```python
from build123d import *

# Parameters (mm, degrees)
EXTRUDE_1_DEPTH     = 20
REVOLVE_1_ANGLE     = 180
CUT_EXTRUDE_START   = -19
CUT_EXTRUDE_1_DEPTH = 19
SKETCH_5_R          = 10
CUT_EXTRUDE_2_DEPTH = 87.442177205
SKETCH_4_R          = 1.25
SKETCH_4_R_2        = 5.1
CUT_EXTRUDE_3_DEPTH = 86.97819491
CUT_EXTRUDE_START_2 = -3
CUT_EXTRUDE_5_DEPTH = 3
SKETCH_6_R          = 6
CUT_EXTRUDE_4_DEPTH = 4.2
CUT_EXTRUDE_6_DEPTH = 5
HOLE_WIZARD_1_D     = 1.7
HOLE_WIZARD_1_DEPTH = 3.5
CHAMFER_1_SIZE      = 0.3


with BuildPart() as part:
    # 草图2 → 凸台-拉伸1 (new body)
    with BuildSketch(Plane(origin=(0, 0, 0), x_dir=(1, 0, 0), z_dir=(0, 1, 0))):
        with BuildLine():
            Line((70.446428571, 12.492025518), (0.535714286, 14.990430621))
            ThreePointArc((0.535714286, 14.990430621), (-10.415476122, 10.794343757), (-15, 0))
            Line((-15, 0), (82.5, 0))
            ThreePointArc((82.5, 0), (78.995286464, 8.679563435), (70.446428571, 12.492025518))
        make_face()
        with BuildLine():
            Line((82.5, 0), (-15, 0))
            ThreePointArc((-15, 0), (-10.415476122, -10.794343757), (0.535714286, -14.990430621))
            Line((0.535714286, -14.990430621), (70.446428571, -12.492025518))
            ThreePointArc((70.446428571, -12.492025518), (78.995286464, -8.679563435), (82.5, 0))
        make_face()
    extrude(amount=EXTRUDE_1_DEPTH)

    # 草图1 → 旋转1 (revolve)
    with BuildSketch(Plane(origin=(0, 0, 0), x_dir=(1, 0, 0), z_dir=(0, 1, 0))):
        with BuildLine():
            Line((0.535714286, -14.990430621), (70.446428571, -12.492025518))
            ThreePointArc((70.446428571, -12.492025518), (78.995286464, -8.679563435), (82.5, 0))
            Line((82.5, 0), (-15, 0))
            ThreePointArc((-15, 0), (-10.415476122, -10.794343757), (0.535714286, -14.990430621))
        make_face()
    revolve(axis=Axis((70, 0, 0), (1, 0, 0)), revolution_arc=REVOLVE_1_ANGLE)

    # 草图3 → 切除-拉伸1 (cut)
    with BuildSketch(Plane(origin=(0, 20, 0), x_dir=(1, 0, 0), z_dir=(0, 1, 0)).offset(CUT_EXTRUDE_START)):
        with BuildLine():
            Line((17.295525226, 14.391483841), (0.535714286, 14.990430621))
            ThreePointArc((0.535714286, 14.990430621), (-15, 0), (0.535714286, -14.990430621))
            Line((0.535714286, -14.990430621), (17.295525226, -14.391483841))
            ThreePointArc((17.295525226, -14.391483841), (22.5, 0), (17.295525226, 14.391483841))
        make_face()
    extrude(amount=CUT_EXTRUDE_1_DEPTH, mode=Mode.SUBTRACT)

    # 草图5 → 切除-拉伸2 (cut, through all)
    with BuildSketch(Plane(origin=(0, -1, 0), x_dir=(1, 0, 0), z_dir=(0, 1, 0))):
        with Locations(Location((0, 0, 0), (0, 0, 270))):
            Circle(SKETCH_5_R)
    extrude(amount=-CUT_EXTRUDE_2_DEPTH, mode=Mode.SUBTRACT)

    # 草图4 → 切除-拉伸3 (cut, through all)
    with BuildSketch(Plane(origin=(0, 1, 0), x_dir=(1, 0, 0), z_dir=(0, 1, 0))):
        with Locations(Location((8, 0, 0), (0, 0, 270))):
            Circle(SKETCH_4_R)
        with Locations(Location((5.656854249, -5.656854249, 0), (0, 0, 270))):
            Circle(SKETCH_4_R)
        with Locations(Location((0, -8, 0), (0, 0, 270))):
            Circle(SKETCH_4_R)
        with Locations(Location((-5.656854249, -5.656854249, 0), (0, 0, 270))):
            Circle(SKETCH_4_R)
        with Locations(Location((-8, 0, 0), (0, 0, 270))):
            Circle(SKETCH_4_R)
        with Locations(Location((-5.656854249, 5.656854249, 0), (0, 0, 270))):
            Circle(SKETCH_4_R)
        with Locations(Location((0, 8, 0), (0, 0, 270))):
            Circle(SKETCH_4_R)
        with Locations(Location((5.656854249, 5.656854249, 0), (0, 0, 270))):
            Circle(SKETCH_4_R)
        with Locations(Location((0, 0, 0), (0, 0, 270))):
            Circle(SKETCH_4_R_2)
    extrude(amount=-CUT_EXTRUDE_3_DEPTH, mode=Mode.SUBTRACT)

    # 草图11 → 切除-拉伸5 (cut)
    with BuildSketch(Plane(origin=(0, 20, 0), x_dir=(1, 0, 0), z_dir=(0, 1, 0)).offset(CUT_EXTRUDE_START_2)):
        with BuildLine():
            Line((60.465308, 12.848721667), (70.446428571, 12.492025518))
            ThreePointArc((70.446428571, 12.492025518), (82.5, 0), (70.446428571, -12.492025518))
            Line((70.446428571, -12.492025518), (60.465308, -12.848721667))
            ThreePointArc((60.465308, -12.848721667), (54, 0), (60.465308, 12.848721667))
        make_face()
    extrude(amount=CUT_EXTRUDE_5_DEPTH, mode=Mode.SUBTRACT)

    # 草图6 → 切除-拉伸4 (cut)
    with BuildSketch(Plane(origin=(0, 17, 0), x_dir=(1, 0, 0), z_dir=(0, 1, 0))):
        with Locations(Location((70, 0, 0), (0, 0, 270))):
            Circle(SKETCH_6_R)
    extrude(amount=-CUT_EXTRUDE_4_DEPTH, mode=Mode.SUBTRACT)

    # 草图12 → 切除-拉伸6 (cut)
    with BuildSketch(Plane(origin=(0, 20, 0), x_dir=(1, 0, 0), z_dir=(0, 1, 0))):
        Polygon((30.581948853, -5.411239688), (30.760520282, -10.408049895), (38.755416613, -10.122335609), (38.576845185, -5.125525402), align=None)
        Polygon((38.576845185, -5.125525402), (38.755416613, -10.122335609), (46.750312944, -9.836621323), (46.571741516, -4.839811116), align=None)
    extrude(amount=-CUT_EXTRUDE_6_DEPTH, mode=Mode.SUBTRACT)

    # 孔1
    with Locations(Plane(origin=(0.535714286, 0, 14.990430621), x_dir=(0.9993620414023731, 0, -0.035714285714285726), z_dir=(0.035714285714285726, 0, 0.9993620414023731))):
        with Locations((35.369180276, 17.5), (41.369180276, 17.5)):
            Hole(HOLE_WIZARD_1_D / 2, depth=HOLE_WIZARD_1_DEPTH)

    # 倒角1
    chamfer_1_edges = [part.edges().sort_by_distance(p)[0] for p in [
        (38.755416613, 20, 10.122335609),
        (46.66102723, 20, 7.33821622),
        (38.576845185, 20, 5.125525402),
        (30.671234568, 20, 7.909644791),
    ]]
    chamfer(chamfer_1_edges, length=CHAMFER_1_SIZE)


solid = part.part
```
The listing builds one solid part. Answer for the finished solid, in the listing's coordinates (mm). A direction names the side the tool comes from. Give positions to 0.01 mm unless a question says otherwise; leave off trailing zeros. Order: outer loops, then holes, each group sorted by start corner. A loop starts at its lowest first (then second) coordinate and runs counter-clockwise, first axis right, second up. Notation, with made-up numbers: (-32.75, 15) -> (-12.75, 15) arc R18 cw to (-12.75, 49) -> close; hole circle Ø1 at (25, 79). An arc over 180 degrees is marked (long way). One line per item, written item: value.
1) Determine the mould class of faces 1 (the conical face through (35.98, -13.72, 0.3)), 2 (the flat face through (39, 20, 0)), 3 (the flat face through (70, 12.8, 0)) for opening direction Z: pulls with the +Z half, pulls with the -Z half, needs draft (parallel to the pull), parting line crosses it, or undercut.
Reported:
face 1: parting line crosses it
face 2: needs draft
face 3: undercut
2) Find section C-C, the plane y = 2. Determine the outline of the cut face in (x, z).
Reported:
outline: (17.3, -14.39) -> (70.45, -12.49) arc R12.5 ccw to (70.45, 12.49) -> (17.3, 14.39) arc R22.5 cw to start
3) Flat-ended cylindrical pins translate along their axes: P1, Ø4, axis at x = 17.5, y = 6, coming from the -Z side; P2, Ø1.5, axis at y = 12, z = 9.5, coming from the +X side; P3, Ø1, axis at x = 63, z = 7.5, coming from the -Y side; P4, Ø5, axis at y = -1, z = -1, coming from the +X side. Find the tip coordinate at first contact, or state that the pin passes through.
Reported:
P1: stops at z = -14.39
P2: stops at x = 78.93
P3: stops at y = -10.67
P4: stops at x = 82.5
4) A tool of negligible diameter and unlimited length cuts with its end or side. For faces 4 (the cylindrical face through (41.03, 17.174, 11.768)), 5 (the flat face through (39, 15, 8)), 6 (the cylindrical face through (22.5, 10.4, 0.2)), 7 (the cylindrical face through (54, 18, 0)), from which of +Z, -Z, +X, -X, +Y, -Y can it reach the whole face along a straight path? Write none if from no direction.
Reported:
face 4: none
face 5: +Y
face 6: -X, +Y
face 7: +X, +Y
5) Find section D-D, the plane x = 8. Determine the outline of the cut face in (y, z), plus the area to 3 significant figures.
Reported:
outline: (-13.45, -6) arc R14.72 ccw to (0, -14.72) -> (1, -14.72) -> (1, -1.25) -> (-1, -1.25) -> (-1, -6) -> close; (-13.45, 6) -> (-1, 6) -> (-1, 1.25) -> (1, 1.25) -> (1, 14.72) -> (0, 14.72) arc R14.72 ccw to start
area: 205 mm^2
6) Find section A-A, the plane x = -8. Determine the outline of the cut face in (y, z), plus the area to 3 significant figures.
Reported:
outline: (-11.18, -6) arc R12.69 ccw to (0, -12.69) -> (1, -12.69) -> (1, -1.25) -> (-1, -1.25) -> (-1, -6) -> close; (-11.18, 6) -> (-1, 6) -> (-1, 1.25) -> (1, 1.25) -> (1, 12.69) -> (0, 12.69) arc R12.69 ccw to start
area: 139 mm^2
7) Find the intervals of material crossed by line 1 (X direction, y = 14, z = -4.5); line 2 (X direction, y = -7, z = -4.5); line 3 (Y direction, x = -6, z = -0.5), in increasing order.
Reported:
line 1: x = 22.05 to 66.03, 73.97 to 81.66
line 2: x = -12.48 to -8.93, 8.93 to 79.33
line 3: y = -1 to 1
8) Find section B-B, the plane x = 71.5. Determine the outline of the cut face in (y, z).
Reported:
outline: (0, -12.41) -> (17, -12.41) -> (17, -5.81) -> (12.8, -5.81) -> (12.8, 5.81) -> (17, 5.81) -> (17, 12.41) -> (0, 12.41) arc R12.41 ccw to start
